For this review, take the finished solid that the model builds, in its own axes (mm). A direction names the side the tool comes from. Round coordinates to 2 decimals unless told otherwise and drop trailing zeros. Loops run counter-clockwise (first coordinate to the right, second up) from the corner with the lowest first, then second, coordinate; pieces in that order, holes last.
Autodesk Inventor part; units mm, degrees
ref_plane "YZ Plane" through (0, 0, 0) normal (1, 0, 0) x (0, 1, 0)
ref_plane "XZ Plane" through (0, 0, 0) normal (0, 1, 0) x (-1, 0, 0)
ref_plane "XY Plane" through (0, 0, 0) normal (0, 0, 1) x (1, 0, 0)
sketch "Sketch1" plane through (0, 0, 0) normal (0, 1, 0) x (-1, 0, 0)
  circle A0 centre (-14.1421, -14.1421) radius 2.5
  circle A1 centre (-14.1421, 14.1421) radius 2.5
  line L0 (0, 0) -> (-14.1421, 14.1421)
  line L1 (0, 0) -> (0, -20)
  line L2 (0, 0) -> (-14.1421, -14.1421)
  circle A2 centre (0, -20) radius 2.5
  circle A3 centre (0, 0) radius 25
  line L3 (0, 0) -> (14.1421, 14.1421)
  line L4 (0, 0) -> (14.1421, -14.1421)
  circle A4 centre (14.1421, 14.1421) radius 2.5
  circle A5 centre (14.1421, -14.1421) radius 2.5
  line L5 (-10, 10) -> (10, 10)
  line L6 (10, 10) -> (10, -10)
  line L7 (10, -10) -> (-10, -10)
  line L8 (-10, -10) -> (-10, 10)
  line L9 (-10, 10) -> (10, -10) construction
  line L10 (10, 10) -> (-10, -10) construction
  dimension "d0" = 20
  dimension "d1" = 20
  dimension "d2" = 135
  dimension "d3" = 5
  dimension "d4" = 5
  dimension "d5" = 20
  dimension "d6" = 90
  dimension "d7" = 5
  dimension "d8" = 20
  dimension "d9" = 90
  dimension "d10" = 5
  dimension "d11" = 20
  dimension "d12" = 90
  dimension "d13" = 5
  dimension "d14" = 20
  dimension "d15" = 20
extrude "Extrusion1" add sketch "Sketch1" along normal blind 10
properties part number "base"
(1) Add section C-C (y = 4.75). Give the boundary of the cut face in (x, z), plus the area to 3 significant figures.
(2) Insertion check: pin 1 Ø6.5 at (x, z) = (0, -20) entering from -Y; pin 2 Ø2 at (x, y) = (-11.5, 1) entering from +Z; pin 3 Ø5 at (x, y) = (2.5, 6) entering from +Z; pin 4 Ø3 at (x, y) = (-18, 4.5) entering from -Z. Each pin has a flat end and moves straight along its axis. Give the tip position at first contact, or say it passes through.
(3) For faces 4 (the flat face through (-10, 5, 0)), 5 (the flat face through (-11, 0, 0)), list the 3-axis set-ups (+Z, -Z, +X, -X, +Y, -Y) from which the entire face can be reached by the end or side of a thin tool; tool diameter is ignored.
(4) Add section B-B (z = 0). Give the boundary of the cut face in (x, y), plus the area to 3 significant figures.
(5) Add section A-A (x = 0). Give the boundary of the cut face in (y, z), plus the area to 3 significant figures.
(6) Add section D-D (x = -8). Give the boundary of the cut face in (y, z).
(7) For L1, parallel to Z at x = 0, y = 4.5; L2, parallel to Z at x = -0.5, y = 2 (3 decimals); L3, parallel to X at y = 4.5, z = 15.5, list the stretches that pass through material, from the lowest coordinate up.
(8) The part is to be moulded in two halves that separate along X. For faces 1 (the flat face through (-11, 10, 0)), 2 (the cylindrical face through (-23.846, 4.93, -7.509)), 3 (the cylindrical face through (12.8, 4.93, -16.25)), say which applies: pulls with the +X half, pulls with the -X half, needs draft (parallel to the pull), parting line crosses it, or undercut.
Outcome:
1. outline: circle Ø50 at (0, 0); hole circle Ø5 at (-14.14, -14.14); hole circle Ø5 at (-14.14, 14.14); hole (-10, -10) - (10, -10) - (10, 10) - (-10, 10) - close; hole circle Ø5 at (0, -20); hole circle Ø5 at (14.14, -14.14); hole circle Ø5 at (14.14, 14.14)
1. area: 1,470 mm2
2. pin 1: stops at y = 0
2. pin 2: stops at z = 22.69
2. pin 3: stops at z = 25
2. pin 4: stops at z = -18.78
3. face 4: +Y, -Y
3. face 5: +Z, -Z, +X, -X, -Y
4. outline: (-25, 0) - (-10, 0) - (-10, 10) - (-25, 10) - close; (10, 0) - (25, 0) - (25, 10) - (10, 10) - close
4. area: 300 mm2
5. outline: (0, -25) - (10, -25) - (10, -22.5) - (0, -22.5) - close; (0, -17.5) - (10, -17.5) - (10, -10) - (0, -10) - close; (0, 10) - (10, 10) - (10, 25) - (0, 25) - close
5. area: 250 mm2
6. outline: (0, -23.69) - (10, -23.69) - (10, -10) - (0, -10) - close; (0, 10) - (10, 10) - (10, 23.69) - (0, 23.69) - close
7. L1: z = -25 to -22.5, -17.5 to -10, 10 to 25
7. L2: z = -24.995 to -22.449, -17.551 to -10, 10 to 24.995
7. L3: x = -19.62 to -16.24, -12.04 to 12.04, 16.24 to 19.62
8. face 1: needs draft
8. face 2: parting line crosses it
8. face 3: undercut
